The drawing under review shows one solid part. Ordinate dimensions are in mm from its lowest x, y, z. A direction names the side the tool comes from. Coordinates: 2 decimals unless noted, no trailing zeros. Write each loop counter-clockwise with the first axis right and the second up, starting at its lowest first coordinate (ties: lowest second). Pieces come first, ordered by that corner, then holes. Notation, with made-up numbers: (65.25, -18) -> (107.25, -18) arc R15 ccw to (107.25, -8) -> close; hole circle Ø2 at (26, -28). An arc over 180 degrees is marked (long way). One line per question, with ' | ' between items. Start each with the question number.
Q1. Add section A-A on x = 114.3. State the section outline as (y, z) points, and give its area (3 significant figures).
Q2. Wall thickness on probe 1 along X at (y, z) = (16, 50); probe 2 along X at (y, z) = (86, 5.5); probe 3 along Z at (x, y) = (114.3, 23): over which ranges is each line inside the solid? List them lowest first.
Q3. Add section B-B on z = 14.5. State the section outline as (x, y) points.
Q4. For the marked faces 1, 2 and 3, list the 3-axis set-ups (+Z, -Z, +X, -X, +Y, -Y) from which the entire face can be reached by the end or side of a thin tool; tool diameter is ignored.
Q5. For P1, Ø20.5, axis at x = 53.5, z = 49, coming from the +Y side; P2, Ø12, axis at x = 50.5, y = 210, coming from the +Z side, all flat-tipped, find the tip position at first contact; note any pin that passes through.
Q6. Add section D-D on x = 29. State the section outline as (y, z) points, and give its area (3 significant figures).
Q7. Add section C-C on y = 236. State the section outline as (x, z) points, and give its area (3 significant figures).
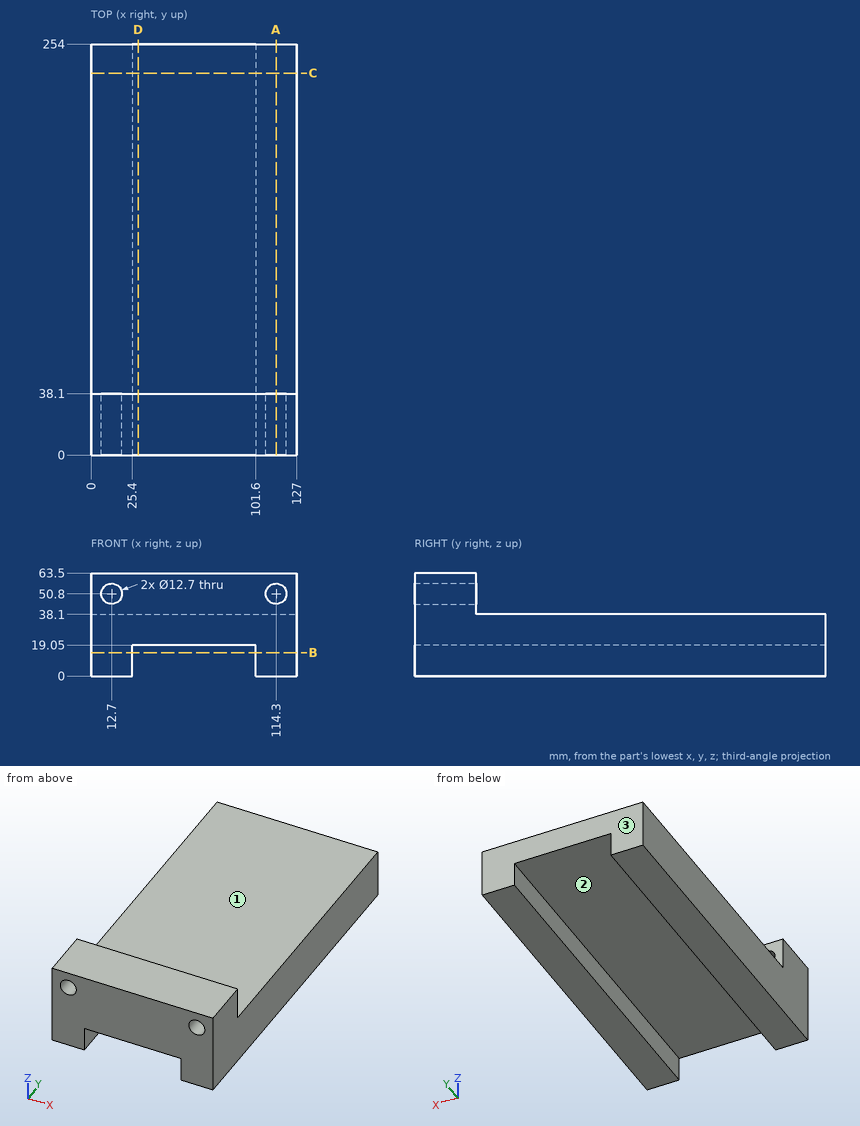
Output values:
1) outline: (0, 0) -> (254, 0) -> (254, 38.1) -> (38.1, 38.1) -> (38.1, 44.45) -> (0, 44.45) -> close; (0, 57.15) -> (38.1, 57.15) -> (38.1, 63.5) -> (0, 63.5) -> close | area: 10,200 mm2
2) probe 1: x = 0 to 6.4, 19 to 108, 120.6 to 127 | probe 2: x = 0 to 25.4, 101.6 to 127 | probe 3: z = 0 to 44.45, 57.15 to 63.5
3) outline: (0, 0) -> (25.4, 0) -> (25.4, 254) -> (0, 254) -> close; (101.6, 0) -> (127, 0) -> (127, 254) -> (101.6, 254) -> close
4) face 1: +Z, +X, -X, +Y | face 2: -Z, +Y, -Y | face 3: +Z, -Z, +X, -X, +Y
5) P1: stops at y = 38.1 | P2: stops at z = 38.1
6) outline: (0, 19.05) -> (254, 19.05) -> (254, 38.1) -> (38.1, 38.1) -> (38.1, 63.5) -> (0, 63.5) -> close | area: 5,810 mm2
7) outline: (0, 0) -> (25.4, 0) -> (25.4, 19.05) -> (101.6, 19.05) -> (101.6, 0) -> (127, 0) -> (127, 38.1) -> (0, 38.1) -> close | area: 3,390 mm2
